from build123d import *

# Parameters (mm, degrees)
F0_W      = 57.15
F0_H      = 6.35
F1_DEPTH  = 38.1
F2_R      = 5.08
F3_W      = 31.75
F3_H      = 38.1
F4_DEPTH  = 12.7
F6_DEPTH  = 25.4
F7_R      = 8.072942
F8_DEPTH  = 25.4
F9_R      = 4.506812
F9_R_2    = 4.48794
F10_DEPTH = 25.4


with BuildPart() as f1:
    # F0 (on Front) → F1 (new body)
    with BuildSketch(Plane.XZ):
        with Locations((28.575, 3.175)):
            Rectangle(F0_W, F0_H)
    extrude(amount=F1_DEPTH)

    # F2
    f2_edges = [f1.edges().sort_by_distance(p)[0] for p in [
        (0, -38.1, 3.175),
        (57.15, -38.1, 3.175),
    ]]
    fillet(f2_edges, radius=F2_R)

    # F3 (on Front) → F4 (join)
    with BuildSketch(Plane.XZ):
        with Locations((15.875, 25.30028)):
            Rectangle(F3_W, F3_H)
    extrude(amount=F4_DEPTH)

    # F5 (on face) → F6 (cut)
    with BuildSketch(Plane.XZ.offset(12.7)):
        with BuildLine():
            Line((28.845884, 38.892605), (28.845884, 10.145596))
            ThreePointArc((28.845884, 10.145596), (29.360416, 7.530471), (31.75, 6.35))
            Line((31.75, 6.35), (31.75, 44.35028))
            Line((31.75, 44.35028), (0, 44.35028))
            Line((0, 44.35028), (0, 38.892605))
            ThreePointArc((0, 38.892605), (14.422942, 44.329867), (28.845884, 38.892605))
        make_face()
    extrude(amount=-F6_DEPTH, mode=Mode.SUBTRACT)

    # F7 (on face) → F8 (cut)
    with BuildSketch(Plane.XZ.offset(12.7)):
        with Locations((14.422942, 29.906925)):
            Circle(F7_R)
    extrude(amount=-F8_DEPTH, mode=Mode.SUBTRACT)

    # F9 (on face) → F10 (cut)
    with BuildSketch(Plane.XY.offset(6.35)):
        with Locations((46.293188, -29.690929)):
            Circle(F9_R)
        with Locations((46.293188, -7.977305)):
            Circle(F9_R)
        with Locations((8.512264, -29.690929)):
            Circle(F9_R_2)
    extrude(amount=-F10_DEPTH, mode=Mode.SUBTRACT)


solid = f1.part
Geometry: final body of the model. Coordinates: model frame, mm. A direction names the side the tool comes from. Give positions to 0.01 mm unless a question says otherwise; leave off trailing zeros. Write each loop counter-clockwise with the first axis right and the second up, starting at its lowest first coordinate (ties: lowest second). Pieces come first, ordered by that corner, then holes. Notation, with made-up numbers: (81, 37.5) -> (90, 37.5) arc R29 cw to (90, 70.5) -> close; hole circle Ø10 at (-10.5, -26). An arc over 180 degrees is marked (long way). Answer as a JSON object with one key per item and string values.
1. Access query for faces 4 (the flat face through (28, -23, 6.35)), 5 (the cylindrical face through (10.925, -25.907, 3.219)), 6 (the flat face through (28.846, -6, 25)). Directions: +Z, -Z, +X, -X, +Y, -Y. A direction counts if a zero-diameter tool reaches every point of the face in a straight line with its end or side. Return the directions, or none.
Ans:
{"face 4": "+Z, +X, -Y", "face 5": "+Z, -Z", "face 6": "+Z, +X, +Y, -Y"}
2. Ray query, probe 1 along Z at (x, y) = (8.5, -14); probe 2 along X at (y, z) = (-2, 33); probe 3 along X at (y, z) = (-2.5, 11.5). Return the intervals inside material, ascending. Write a range as from..to.
Ans:
{"probe 1": "z = 0..6.35", "probe 2": "x = 0..6.97, 21.88..28.85", "probe 3": "x = 0..28.85"}
3. Mould query, pull axis Y, two halves, no side actions, for faces 1 (the flat face through (16, -12.7, 21)), 2 (the cylindrical face through (43, -4.9, 3.2)), 3 (the flat face through (57.15, -16, 3)). Classes: pulls with the +Y half, pulls with the -Y half, needs draft (parallel to the pull), parting line crosses it, or undercut.
Ans:
{"face 1": "pulls with the -Y half", "face 2": "undercut", "face 3": "needs draft"}
4. Cut plane D-D on x = 45. Output: boundary loops of the cut face in (y, z), and give its area (3 significant figures).
Ans:
{"outline": "(-38.1, 0) -> (-34.01, 0) -> (-34.01, 6.35) -> (-38.1, 6.35) -> close; (-25.37, 0) -> (-12.29, 0) -> (-12.29, 6.35) -> (-25.37, 6.35) -> close; (-3.66, 0) -> (0, 0) -> (0, 6.35) -> (-3.66, 6.35) -> close", "area": "132 mm^2"}
5. Cut plane B-B on z = 31.5. Output: boundary loops of the cut face in (x, y).
Ans:
{"outline": "(0, -12.7) -> (6.51, -12.7) -> (6.51, 0) -> (0, 0) -> close; (22.34, -12.7) -> (28.85, -12.7) -> (28.85, 0) -> (22.34, 0) -> close"}
6. Cut plane A-A on y = -11. Output: boundary loops of the cut face in (x, z).
Ans:
{"outline": "(0, 0) -> (42.95, 0) -> (42.95, 6.35) -> (31.75, 6.35) arc R3.01 cw to (28.85, 10.15) -> (28.85, 38.89) arc R21.85 ccw to (0, 38.89) -> close; (49.64, 0) -> (57.15, 0) -> (57.15, 6.35) -> (49.64, 6.35) -> close; hole circle Ø16.15 at (14.42, 29.91)"}
7. Contact query for flat-ended pins moving along their axis: pin 1 (10.5 mm diameter, centred on x = 46.29, y = -7.98, fed in from +Z); pin 2 (19 mm diameter, centred on x = 16, y = -23, fed in from +Z); pin 3 (4 mm diameter, centred on y = -3.5, z = 30.5, fed in from +X); pin 4 (8 mm diameter, centred on y = -18.5, z = 37, fed in from +X). Output: stop coordinate, or through.
Ans:
{"pin 1": "stops at z = 6.35", "pin 2": "stops at z = 6.35", "pin 3": "stops at x = 28.85", "pin 4": "passes through"}
8. Cut plane C-C on y = -26. Output: boundary loops of the cut face in (x, z), and give its area (3 significant figures).
Ans:
{"outline": "(0, 0) -> (5.96, 0) -> (5.96, 6.35) -> (0, 6.35) -> close; (11.07, 0) -> (43.71, 0) -> (43.71, 6.35) -> (11.07, 6.35) -> close; (48.88, 0) -> (57.15, 0) -> (57.15, 6.35) -> (48.88, 6.35) -> close", "area": "298 mm^2"}
